The listing builds one solid part. Answer for the finished solid, in the listing's coordinates (mm). A direction names the side the tool comes from. Round coordinates to 2 decimals unless told otherwise and drop trailing zeros. Loops run counter-clockwise (first coordinate to the right, second up) from the corner with the lowest first, then second, coordinate; pieces in that order, holes last. Notation, with made-up numbers: (-9, -24) -> (3, -24) arc R28 ccw to (3, 10) -> close; hole circle Ø1 at (-33.5, 67.25). An arc over 180 degrees is marked (long way). One line per question, with ' | ' between items.
from build123d import *

# Parameters (mm, degrees)
BOSS_EXTRUDE1_DEPTH = 45.9
BOSS_EXTRUDE2_START = 5.85
BOSS_EXTRUDE2_DEPTH = 5.85
SKETCH5_R           = 13
CUT_EXTRUDE1_DEPTH  = 107.896512669
BOSS_EXTRUDE3_DEPTH = 16
CUT_EXTRUDE3_DEPTH  = 108.63296159
FILLET2_R           = 9
SKETCH6_R           = 4.2
CUT_EXTRUDE2_DEPTH  = 148.343120723
SKETCH9_R           = 1.65
CUT_EXTRUDE5_DEPTH  = 107.896512669
CIRPATTERN1_COUNT   = 4
CUT_EXTRUDE6_DEPTH  = 145.539121778
CHAMFER1_SIZE       = 0.5


with BuildPart() as part:
    # Sketch2 → Boss-Extrude1 (new body)
    with BuildSketch(Plane(origin=(0, 0, 0), x_dir=(0, 0, -1), z_dir=(1, 0, 0))):
        with BuildLine():
            Line((-75.607591408, 29.531476198), (-75.607591408, 37.281476198))
            Line((-75.607591408, 37.281476198), (-85.507591408, 37.281476198))
            Line((-85.507591408, 37.281476198), (-85.507591408, 80.281476198))
            Line((-85.507591408, 80.281476198), (-75.607591408, 80.281476198))
            Line((-75.607591408, 80.281476198), (-75.607591408, 88.031476198))
            ThreePointArc((-75.607591408, 88.031476198), (-77.950737158, 93.688330447), (-83.607591408, 96.031476198))
            Line((-83.607591408, 96.031476198), (-91.607591408, 96.031476198))
            Line((-91.607591408, 96.031476198), (-91.607591408, 21.531476198))
            Line((-91.607591408, 21.531476198), (-83.607591408, 21.531476198))
            ThreePointArc((-83.607591408, 21.531476198), (-77.950737158, 23.874621948), (-75.607591408, 29.531476198))
        make_face()
    extrude(amount=BOSS_EXTRUDE1_DEPTH)

    # Sketch3 → Boss-Extrude2 (add)
    with BuildSketch(Plane.ZY.offset(BOSS_EXTRUDE2_START)):
        with BuildLine():
            Line((75.607591408, 37.281476198), (75.607591408, 80.281476198))
            Line((75.607591408, 80.281476198), (75.607591408, 88.031476198))
            ThreePointArc((75.607591408, 88.031476198), (77.950737158, 93.688330447), (83.607591408, 96.031476198))
            Line((83.607591408, 96.031476198), (91.607591408, 96.031476198))
            Line((91.607591408, 96.031476198), (91.607591408, 21.531476198))
            Line((91.607591408, 21.531476198), (83.607591408, 21.531476198))
            ThreePointArc((83.607591408, 21.531476198), (77.950737158, 23.874621948), (75.607591408, 29.531476198))
            Line((75.607591408, 29.531476198), (75.607591408, 37.281476198))
        make_face()
    extrude(amount=-BOSS_EXTRUDE2_DEPTH)

    # Sketch5 → Cut-Extrude1 (cut, through all)
    with BuildSketch(Plane(origin=(0, 0, 85.507591408), x_dir=(-1, 0, 0), z_dir=(0, 0, -1))):
        with Locations(Location((-20.9, 58.781476198, 0), (0, 0, 90))):
            Circle(SKETCH5_R)
    extrude(amount=-CUT_EXTRUDE1_DEPTH, mode=Mode.SUBTRACT)

    # Sketch7 → Boss-Extrude3 (add)
    with BuildSketch(Plane(origin=(0, 0, 75.607591408), x_dir=(-1, 0, 0), z_dir=(0, 0, -1))):
        with BuildLine():
            ThreePointArc((5.85, 50.388771032), (14.186747487, 51.356854995), (18.1, 58.781476198))
            Line((18.1, 58.781476198), (18.1, 96.031476198))
            Line((18.1, 96.031476198), (11.35, 96.031476198))
            Line((11.35, 96.031476198), (11.35, 62.327953323))
            ThreePointArc((11.35, 62.327953323), (12.243437264, 55.996013549), (5.85, 56.121119079))
            Line((5.85, 56.121119079), (5.85, 50.388771032))
        make_face()
    extrude(amount=-BOSS_EXTRUDE3_DEPTH)

    # Sketch7<3> → Cut-Extrude3 (cut, through all)
    with BuildSketch(Plane(origin=(0, 0, 75.607591408), x_dir=(-1, 0, 0), z_dir=(0, 0, -1))):
        with BuildLine():
            ThreePointArc((5.85, 61.441833317), (4.9, 58.781476198), (5.85, 56.121119079))
            Line((5.85, 56.121119079), (5.85, 61.441833317))
        make_face()
    extrude(amount=-CUT_EXTRUDE3_DEPTH, mode=Mode.SUBTRACT)

    # Fillet2
    fillet2_edges = [part.edges().sort_by_distance(p)[0] for p in [
        (-5.85, 50.388771032, 83.607591408),
    ]]
    fillet(fillet2_edges, radius=FILLET2_R)

    # Sketch6 → Cut-Extrude2 (cut, through all)
    with BuildSketch(Plane(origin=(45.9, 0, 0), x_dir=(0, 0, -1), z_dir=(1, 0, 0))):
        with Locations((-83.607591408, 88.031476198)):
            Circle(SKETCH6_R)
        with Locations((-83.607591408, 29.531476198)):
            Circle(SKETCH6_R)
    extrude(amount=-CUT_EXTRUDE2_DEPTH, mode=Mode.SUBTRACT)

    # Sketch9 → Cut-Extrude5 (cut, through all)
    with BuildSketch(Plane(origin=(0, 0, 85.507591408), x_dir=(-1, 0, 0), z_dir=(0, 0, -1))):
        with Locations(Location((-36.4, 74.281476198, 0), (0, 0, 90))):
            Circle(SKETCH9_R)
    cut_extrude5 = extrude(amount=-CUT_EXTRUDE5_DEPTH, mode=Mode.SUBTRACT)

    # CirPattern1: Cut-Extrude5 ×4 about axis
    cirpattern1_axis = Axis((20.9, 58.781476198, 0), (0, 0, 1))
    for i in range(1, CIRPATTERN1_COUNT):
        add(cut_extrude5.rotate(cirpattern1_axis, i * 360 / CIRPATTERN1_COUNT), mode=Mode.SUBTRACT)

    # Sketch10 → Cut-Extrude6 (cut, through all)
    with BuildSketch(Plane(origin=(-11.35, 0, 0), x_dir=(0, 0, -1), z_dir=(1, 0, 0))):
        with BuildLine():
            ThreePointArc((-83.607591408, 96.031476198), (-77.950737158, 93.688330447), (-75.607591408, 88.031476198))
            Line((-75.607591408, 88.031476198), (-75.607591408, 96.031476198))
            Line((-75.607591408, 96.031476198), (-83.607591408, 96.031476198))
        make_face()
    extrude(amount=-CUT_EXTRUDE6_DEPTH, mode=Mode.SUBTRACT)

    # Chamfer1
    chamfer1_edges = [part.edges().sort_by_distance(p)[0] for p in [
        (36.4, 72.631476198, 91.607591408),
        (34.75, 43.281476198, 91.607591408),
        (5.4, 44.931476198, 91.607591408),
        (7.05, 74.281476198, 91.607591408),
        (20.025, 21.531476198, 91.607591408),
        (20.025, 96.031476198, 91.607591408),
        (45.9, 58.781476198, 91.607591408),
        (-5.85, 31.628031146, 91.607591408),
        (20.9, 45.781476198, 91.607591408),
        (-12.243437264, 55.996013549, 91.607591408),
        (-14.725, 96.031476198, 91.607591408),
        (-11.35, 79.17971476, 91.607591408),
        (-18.1, 77.406476198, 91.607591408),
        (-16.410095759, 53.531476198, 91.607591408),
        (-5.85, 78.736654757, 91.607591408),
        (-7.539904241, 46.974586094, 91.607591408),
    ]]
    chamfer(chamfer1_edges, length=CHAMFER1_SIZE)


solid = part.part
Q1. Find the intervals of material crossed by line 1 (Y direction, x = 5.4, z = 88.6); line 2 (X direction, y = 83.5, z = 77.75); line 3 (Y direction, x = 11.5, z = 80), in increasing order. Write a range as from..to.
Numbers:
line 1: 21.53..41.63, 44.93..72.63, 75.93..96.03 | line 2: -18.1..-11.35, -5.85..45.9 | line 3: 22.39..27.38, 31.68..37.28, 80.28..85.88, 90.18..95.17
Q2. A cutting plane is placed at B-B on x = 36.4. Give the vertices of the cut face in (y, z).
Numbers:
outline: (21.53, 83.61) arc R8 ccw to (29.53, 75.61) -> (37.28, 75.61) -> (37.28, 85.51) -> (41.63, 85.51) -> (41.63, 91.11) -> (41.13, 91.61) -> (22.03, 91.61) -> (21.53, 91.11) -> close; (44.93, 85.51) -> (72.63, 85.51) -> (72.63, 91.11) -> (72.13, 91.61) -> (45.43, 91.61) -> (44.93, 91.11) -> close; (75.93, 85.51) -> (80.28, 85.51) -> (80.28, 75.61) -> (88.03, 75.61) arc R8 ccw to (96.03, 83.61) -> (96.03, 91.11) -> (95.53, 91.61) -> (76.43, 91.61) -> (75.93, 91.11) -> close; hole circle Ø8.4 at (29.53, 83.61); hole circle Ø8.4 at (88.03, 83.61)
Q3. A cutting plane is placed at D-D on z = 90. Give the vertices of the cut face in (x, y) (3 decimals).
Numbers:
outline: (-18.1, 58.781) arc R9 ccw to (-11.975, 50.253) arc R9 cw to (-5.85, 41.725) -> (-5.85, 21.531) -> (45.9, 21.531) -> (45.9, 96.031) -> (-5.85, 96.031) -> (-5.85, 61.442) arc R4.2 cw (long way) to (-11.35, 62.328) -> (-11.35, 96.031) -> (-18.1, 96.031) -> close; hole circle Ø3.3 at (5.4, 43.281); hole circle Ø3.3 at (5.4, 74.281); hole circle Ø26 at (20.9, 58.781); hole circle Ø3.3 at (36.4, 43.281); hole circle Ø3.3 at (36.4, 74.281)
Q4. For faces 1 (the face through (-5.85, 34, 83)), 2 (the face through (20, 96.031, 87)), 3 (the face through (0, 59, 81)), determine the directions among +Z, -Z, +X, -X, +Y, -Y from which every point of the face is accessible in a straight line to the end or side of a thin tool.
Numbers:
face 1: +Z, -Z, -X, -Y | face 2: +Z, -Z, +X, -X, +Y | face 3: -Z, +X
Q5. For a pull along Z with two mould halves and no side action, classify faces 4 (the face through (-14.68, 83.93, 84.52)), 5 (the face through (33, 68, 85.508)), 6 (the face through (6, 59, 91.608)), 7 (the face through (-5.85, 79, 83)) as pulls with the +Z half, pulls with the -Z half, needs draft (parallel to the pull), parting line crosses it, or undercut.
Numbers:
face 4: undercut | face 5: pulls with the -Z half | face 6: pulls with the +Z half | face 7: needs draft
Q6. A cutting plane is placed at A-A on x = 20.9. Give the vertices of the cut face in (y, z), plus the area to 3 significant figures.
Numbers:
outline: (21.53, 83.61) arc R8 ccw to (29.53, 75.61) -> (37.28, 75.61) -> (37.28, 85.51) -> (45.78, 85.51) -> (45.78, 91.11) -> (45.28, 91.61) -> (22.03, 91.61) -> (21.53, 91.11) -> close; (71.78, 85.51) -> (80.28, 85.51) -> (80.28, 75.61) -> (88.03, 75.61) arc R8 ccw to (96.03, 83.61) -> (96.03, 91.11) -> (95.53, 91.61) -> (72.28, 91.61) -> (71.78, 91.11) -> close; hole circle Ø8.4 at (29.53, 83.61); hole circle Ø8.4 at (88.03, 83.61) | area: 469 mm^2
Q7. Given pin 1 Ø5.5 at (x, y) = (5.4, 43.28) entering from -Z; pin 2 Ø3 at (x, z) = (25, 81) entering from -Y; pin 3 Ø6 at (y, z) = (54.5, 87) entering from -X, each flat-ended and moving along its own axis, determine where each tip first touches the part or whether it passes through.
Numbers:
pin 1: z = 85.51 | pin 2: y = 21.61 | pin 3: x = -18.01
Q8. A cutting plane is placed at C-C on y = 89. Give the vertices of the cut face in (x, z), plus the area to 3 significant figures.
Numbers:
outline: (-18.1, 75.67) -> (-11.35, 75.67) -> (-11.35, 79.52) -> (-18.1, 79.52) -> close; (-18.1, 87.69) -> (-11.35, 87.69) -> (-11.35, 91.11) -> (-11.85, 91.61) -> (-17.6, 91.61) -> (-18.1, 91.11) -> close; (-5.85, 75.67) -> (45.9, 75.67) -> (45.9, 79.52) -> (-5.85, 79.52) -> close; (-5.85, 87.69) -> (45.9, 87.69) -> (45.9, 91.11) -> (45.4, 91.61) -> (-5.35, 91.61) -> (-5.85, 91.11) -> close | area: 454 mm^2
